```python
from build123d import *

# Parameters (mm, degrees)
F0_W     = 101.6
F0_H     = 63.5
F1_DEPTH = 31.75
F2_R     = 5.08
F3_R     = 12.7
F4_DEPTH = 86.868
F4_TAPER = -3
F5_R     = 2.54


with BuildPart() as f1:
    # F0 (on Top) → F1 (new body, symmetric)
    with BuildSketch(Plane.XY):
        Rectangle(F0_W, F0_H)
    extrude(amount=F1_DEPTH, both=True)

    # F2
    f2_edges = [f1.edges().sort_by_distance(p)[0] for p in [
        (50.8, 0, 31.75),
        (0, 31.75, 31.75),
        (-50.8, 0, 31.75),
        (0, -31.75, 31.75),
        (0, -31.75, -31.75),
        (50.8, -31.75, 0),
        (-50.8, -31.75, 0),
        (-50.8, 31.75, 0),
        (-50.8, 0, -31.75),
        (50.8, 0, -31.75),
        (0, 31.75, -31.75),
        (50.8, 31.75, 0),
    ]]
    fillet(f2_edges, radius=F2_R)

    # F3 (on face) → F4 (cut)
    with BuildSketch(Plane.XY.offset(31.75)):
        Circle(F3_R)
    extrude(amount=-F4_DEPTH, taper=F4_TAPER, mode=Mode.SUBTRACT)

    # F5
    f5_edges = [f1.edges().sort_by_distance(p)[0] for p in [
        (-12.7, 0, 31.75),
        (-16.027894, 0, -31.75),
    ]]
    fillet(f5_edges, radius=F5_R)


solid = f1.part
```
Model file for the job. Use its own axes, mm. Coordinates: 2 decimals unless noted, no trailing zeros. Write each loop counter-clockwise with the first axis right and the second up, starting at its lowest first coordinate (ties: lowest second). Pieces come first, ordered by that corner, then holes. Notation, with made-up numbers: (49, 69) - (105, 69) arc R28 cw to (105, 94) - close; hole circle Ø1 at (56.25, 26). An arc over 180 degrees is marked (long way). Use a Markdown table: item, result. Add a question column.
Item 1: Drill centre lines: line 1 along X through (y, z) = (-2.5, 16); line 2 along Y through (x, z) = (-7, -19); line 3 along Z through (x, y) = (-42.5, 27). Where is each one in solid material? Low to high.
Item 2: Two-plate mould, pull along Y, no slides. Class faces 1 (the face through (-49.351, 0.373, -30.222)), 2 (the face through (7.737, 12.136, -0.542)), 3 (the face through (49.351, -30.222, 0.373)), 4 (the face through (0.64, 30.222, 30.301)): pulls with the +Y half, pulls with the -Y half, needs draft (parallel to the pull), parting line crosses it, or undercut.
Item 3: Band-saw the part on A-A, the plane z = -9.5. Write the cut outline in (x, y), and give its area (3 significant figures).
Item 4: Band-saw the part on B-B, the plane x = 0. Write the cut outline in (y, z).
Item 5: Band-saw the part on C-C, the plane z = -17. Write the cut outline in (x, y), and give its area (3 significant figures).
A:
| question | item | result |
|---|---|---|
| 1 | line 1 | x = -50.8 to -13.29, 13.29 to 50.8 |
| 1 | line 2 | y = -31.75 to -13.67, 13.67 to 31.75 |
| 1 | line 3 | z = -31.74 to 31.74 |
| 2 | face 1 | needs draft |
| 2 | face 2 | undercut |
| 2 | face 3 | pulls with the -Y half |
| 2 | face 4 | pulls with the +Y half |
| 3 | outline | (-50.8, -26.67) arc R5.08 ccw to (-45.72, -31.75) - (45.72, -31.75) arc R5.08 ccw to (50.8, -26.67) - (50.8, 26.67) arc R5.08 ccw to (45.72, 31.75) - (-45.72, 31.75) arc R5.08 ccw to (-50.8, 26.67) - close; hole circle Ø29.72 at (0, 0) |
| 3 | area | 5,740 mm² |
| 4 | outline | (-31.75, -26.67) arc R5.08 ccw to (-26.67, -31.75) - (-18.44, -31.75) arc R2.54 ccw to (-15.9, -29.34) - (-12.84, 29.08) arc R2.54 ccw to (-15.38, 31.75) - (-26.67, 31.75) arc R5.08 ccw to (-31.75, 26.67) - close; (12.84, 29.08) - (15.9, -29.34) arc R2.54 ccw to (18.44, -31.75) - (26.67, -31.75) arc R5.08 ccw to (31.75, -26.67) - (31.75, 26.67) arc R5.08 ccw to (26.67, 31.75) - (15.38, 31.75) arc R2.54 ccw to start |
| 5 | outline | (-50.8, -26.67) arc R5.08 ccw to (-45.72, -31.75) - (45.72, -31.75) arc R5.08 ccw to (50.8, -26.67) - (50.8, 26.67) arc R5.08 ccw to (45.72, 31.75) - (-45.72, 31.75) arc R5.08 ccw to (-50.8, 26.67) - close; hole circle Ø30.51 at (0, 0) |
| 5 | area | 5,700 mm² |
